from build123d import *

# Parameters (mm, degrees)
SKETCH1_R           = 3.5
BOSS_EXTRUDE1_DEPTH = 4
SKETCH2_R           = 2.5
CUT_EXTRUDE1_DEPTH  = 2
SKETCH3_R           = 2
BOSS_EXTRUDE2_DEPTH = 1.5


with BuildPart() as part:
    # Sketch1 → Boss-Extrude1 (new body)
    with BuildSketch(Plane(origin=(0, 0, 0), x_dir=(1, 0, 0), z_dir=(0, 1, 0))):
        with Locations(Location((0, 0, 0), (0, 0, 270))):
            Circle(SKETCH1_R)
    extrude(amount=BOSS_EXTRUDE1_DEPTH)

    # Sketch2 → Cut-Extrude1 (cut)
    with BuildSketch(Plane(origin=(0, 4, 0), x_dir=(1, 0, 0), z_dir=(0, 1, 0))):
        with Locations(Location((0, 0, 0), (0, 0, 270))):
            Circle(SKETCH2_R)
    extrude(amount=-CUT_EXTRUDE1_DEPTH, mode=Mode.SUBTRACT)

    # Sketch3 → Boss-Extrude2 (add)
    with BuildSketch(Plane(origin=(0, 0, 0), x_dir=(1, 0, 0), z_dir=(0, 1, 0))):
        with Locations((16, 0)):
            Circle(SKETCH3_R)
        with BuildLine():
            Line((16, 2), (0.65053243, 3.439012585))
            ThreePointArc((0.65053243, 3.439012585), (2.695075463, 2.233062527), (3.5, 0))
            ThreePointArc((3.5, 0), (2.695075463, -2.233062527), (0.65053243, -3.439012585))
            Line((0.65053243, -3.439012585), (16, -2))
            ThreePointArc((16, -2), (14, 0), (16, 2))
        make_face()
    extrude(amount=BOSS_EXTRUDE2_DEPTH)


solid = part.part
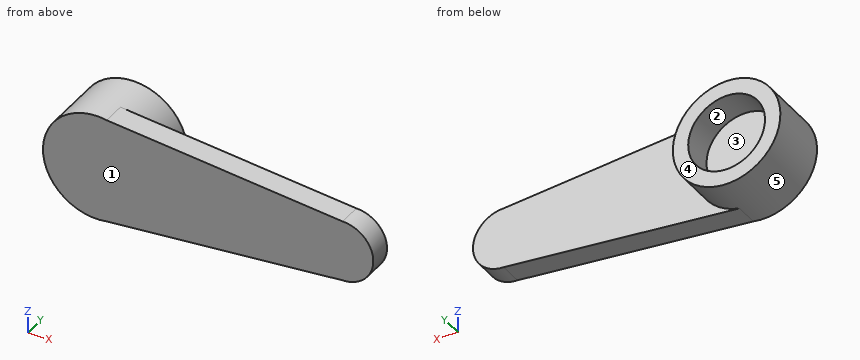
Geometry: final body of the model. Coordinates: model frame, mm. Face numbers are marked on the shaded views. A direction names the side the tool comes from. Coordinates: 2 decimals unless noted, no trailing zeros. Loops run counter-clockwise (first coordinate to the right, second up) from the corner with the lowest first, then second, coordinate; pieces in that order, holes last. Notation, with made-up numbers: M 67,65 L 99,65 A4 ccw 99,71 Z; hole C -17,31 d2. An arc over 180 degrees is marked long. One line per item, written item: value. Start each with the question number.
1) Cut plane B-B (y = 3.45). Return loops of the section in (x, z), then the cut area to 3 significant figures.
2) Pin query (flat end, axial travel): P1, Ø1.5, axis at x = 11, y = 1, coming from the +Z side; P2, Ø1.5, axis at x = 6, y = 2, coming from the +Z side; P3, Ø1, axis at x = 3.5, y = 1.5, coming from the -Z side. Return the tip coordinate at first contact, or that it passes through.
3) Cut plane C-C (x = 0). Return loops of the section in (y, z), then the cut area to 3 significant figures.
4) Cut plane A-A (z = 0). Return loops of the section in (x, y), then the cut area to 4 significant figures.
5) Material intervals for L1, parallel to X at y = 2.9, z = 0; L2, parallel to Y at x = -1.25, z = 0.5; L3, parallel to Y at x = 13.25, z = 0, sorted ascending. Write a range as from..to.
6) Draft query along X for the marked faces 3, 4 and 5. Return one class per face: released by +X, released by -X, zero draft, split by the parting line, or undercut.
7) Reachability of the marked faces 1 and 2 from +Z, -Z, +X, -X, +Y, -Y: full face, straight path, thin tool, end or side. Return the list, or none.
8) Cut plane D-D (y = 0.9). Return loops of the section in (x, z).
Evaluation:
1. outline: C 0,0 d7; hole C 0,0 d5
1. area: 18.8 mm^2
2. P1: z = 2.54
2. P2: z = 2.99
2. P3: z = -3.22
3. outline: M 0,-3.5 L 4,-3.5 L 4,-2.5 L 2,-2.5 L 2,2.5 L 4,2.5 L 4,3.5 L 0,3.5 Z
3. area: 18.0 mm^2
4. outline: M -3.5,0 L 18,0 L 18,1.5 L 3.5,1.5 L 3.5,4 L 2.5,4 L 2.5,2 L -2.5,2 L -2.5,4 L -3.5,4 Z
4. area: 39.75 mm^2
5. L1: -3.5..-2.5, 2.5..3.5
5. L2: 0..2
5. L3: 0..1.5
6. face 3: undercut
6. face 4: zero draft
6. face 5: split by the parting line
7. face 1: +Z, -Z, +X, -X, -Y
7. face 2: +Y
8. outline: M 0.65,-3.44 L 16,-2 A2 ccw 16,2 L 0.65,3.44 A3.5 ccw long Z
